```python
from build123d import *

# Parameters (mm, degrees)
PAD020_DEPTH    = 20
SKETCH071_R     = 4.2
HOLE011_DEPTH   = 25
SKETCH072_R     = 2.75
HOLE012_DEPTH   = 25
SKETCH073_W     = 40
SKETCH073_H     = 20
POCKET025_DEPTH = 10
SKETCH074_W     = 25
SKETCH074_H     = 10
POCKET026_DEPTH = 190.001
SKETCH075_W     = 40
SKETCH075_H     = 10
PAD021_DEPTH    = 2


with BuildPart() as part:
    # Sketch070 → Pad020 (new body)
    with BuildSketch(Plane.XY.offset(480)):
        Polygon((-190, 160), (-190, 140), (-150, 140), (-150, 160), (-150, 194), (-190, 194), align=None)
    extrude(amount=PAD020_DEPTH)

    # Sketch071 (on Face8 of Pad020) → Hole011 (cut)
    with BuildSketch(Plane.XY.offset(500)):
        with Locations((-170, 181)):
            Circle(SKETCH071_R)
    extrude(amount=-HOLE011_DEPTH, mode=Mode.SUBTRACT)

    # Sketch072 (on Face5 of Hole011) → Hole012 (cut)
    with BuildSketch(Plane.XY.offset(500)):
        with Locations((-180, 150)):
            Circle(SKETCH072_R)
        with Locations((-160, 150)):
            Circle(SKETCH072_R)
    extrude(amount=-HOLE012_DEPTH, mode=Mode.SUBTRACT)

    # Sketch073 (on Face5 of Hole012) → Pocket025 (cut)
    with BuildSketch(Plane.XY.offset(500)):
        with Locations((-170, 150)):
            Rectangle(SKETCH073_W, SKETCH073_H)
    extrude(amount=-POCKET025_DEPTH, mode=Mode.SUBTRACT)

    # Sketch074 → Pocket026 (cut, through all)
    with BuildSketch(Plane.YZ):
        with Locations((181.5, 485)):
            Rectangle(SKETCH074_W, SKETCH074_H)
    extrude(amount=-POCKET026_DEPTH, mode=Mode.SUBTRACT)

    # Sketch075 (on Face13 of Pocket026) → Pad021 (join)
    with BuildSketch(Plane.XY.offset(500)):
        with Locations((-170, 181)):
            Rectangle(SKETCH075_W, SKETCH075_H)
    extrude(amount=PAD021_DEPTH)


solid = part.part
```
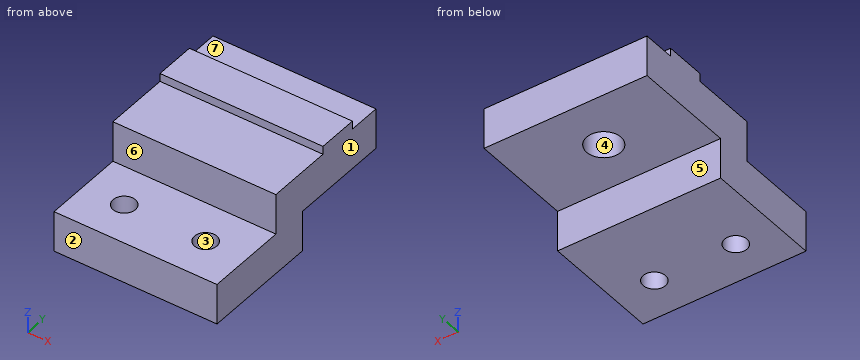
Geometry check sheet. Reference: the model listing, model coordinates, mm. Face numbers are marked on the shaded views. A direction names the side the tool comes from. Coordinates: 2 decimals unless noted, no trailing zeros. Order: outer loops, then holes, each group sorted by start corner. A loop starts at its lowest first (then second) coordinate and runs counter-clockwise, first axis right, second up. Notation, with made-up numbers: M 12,73.25 L 37,73.25 A14 ccw 37,100.25 Z; hole C 43,36 d2. An arc over 180 degrees is marked long. One line per question, with ' | ' between items. Start each with the question number.
Item 1: Cross-section at B-B on x = -160. Enter the section's corners in (y, z).
Item 2: Cross-section at C-C on z = 489. Enter the section's corners in (x, y).
Item 3: Draft check along X on the marked faces 1, 2 and 3. Enter one of: pulls with the +X half, pulls with the -X half, needs draft (parallel to the pull), parting line crosses it, or undercut.
Item 4: Gauge pin test, flat ends, axial feed: pin 1 (0.6 mm diameter, centred on x = -174.5, z = 501, fed in from +Y); pin 2 (2.5 mm diameter, centred on x = -168, y = 182, fed in from -Z); pin 3 (16 mm diameter, centred on x = -163, y = 151.5, fed in from +Z). Record the tip position at first contact, or that the pin passes through.
Item 5: Set-up check for the marked faces 4, 5, 6 and 7: record each of +Z, -Z, +X, -X, +Y, -Y from which the full face is reachable in a straight line by a thin tool's end or side.
Item 6: Cross-section at D-D on y = 181. Enter the section's corners in (x, z).
Item 7: Material ranges on L1, parallel to X at y = 150, z = 485.75; L2, parallel to Y at x = -160, z = 486.5; L3, parallel to Y at x = -170, z = 497.5, recorded low to high. Write a range as [from, to].
Item 8: Cross-section at A-A on y = 150. Enter the section's corners in (x, z), then the cut area to 3 significant figures.
Findings:
1) outline: M 140,480 L 147.25,480 L 147.25,490 L 140,490 Z; M 152.75,480 L 169,480 L 169,490 L 194,490 L 194,500 L 186,500 L 186,502 L 176,502 L 176,500 L 160,500 L 160,490 L 152.75,490 Z
2) outline: M -190,140 L -150,140 L -150,169 L -190,169 Z; hole C -180,150 d5.5; hole C -160,150 d5.5
3) face 1: pulls with the +X half | face 2: needs draft | face 3: undercut
4) pin 1: stops at y = 186 | pin 2: stops at z = 500 | pin 3: stops at z = 490
5) face 4: -Z | face 5: -Z, +X, -X, +Y | face 6: +Z, +X, -X, -Y | face 7: +Z, +X, -X, +Y
6) outline: M -190,490 L -174.2,490 L -174.2,500 L -165.8,500 L -165.8,490 L -150,490 L -150,502 L -190,502 Z
7) L1: x = [-190, -182.75], [-177.25, -162.75], [-157.25, -150] | L2: y = [140, 147.25], [152.75, 169] | L3: y = [160, 176.8], [185.2, 194]
8) outline: M -190,480 L -182.75,480 L -182.75,490 L -190,490 Z; M -177.25,480 L -162.75,480 L -162.75,490 L -177.25,490 Z; M -157.25,480 L -150,480 L -150,490 L -157.25,490 Z | area: 290 mm²
